For this review, take the finished solid that the model builds, in its own axes (mm). Face numbers are marked on the shaded views. A direction names the side the tool comes from. Give positions to 0.01 mm unless a question says otherwise; leave off trailing zeros. Loops run counter-clockwise (first coordinate to the right, second up) from the corner with the lowest first, then second, coordinate; pieces in that order, holes last. Notation, with made-up numbers: (-21, 22) - (-2, 22) arc R3 ccw to (-2, 26) - close; hole circle Ø7 at (-38, -37.75). An arc over 180 degrees is marked (long way). Answer as CSV lines item,"result".
from build123d import *

# Parameters (mm, degrees)
F0_W      = 50
F0_H      = 30
F1_DEPTH  = 40
F2_W      = 10
F2_H      = 23
F3_DEPTH  = 40.001
F5_DEPTH  = 7.001
F7_DEPTH  = 40.001
F8_DEPTH  = 91
F10_DEPTH = 40.001


# Not quite as in the source:
# - an extrude ends at something that could not be found from the text; its depth is read off the source's solid


with BuildPart() as f1:
    # F0 (on Front) → F1 (new body)
    with BuildSketch(Plane.XZ):
        Rectangle(F0_W, F0_H)
    extrude(amount=F1_DEPTH)

    # F2 (on face) → F3 (cut, through all)
    with BuildSketch(Plane.XZ.offset(40)):
        with Locations((-20, 3.5)):
            Rectangle(F2_W, F2_H)
        with Locations((20, 3.5)):
            Rectangle(F2_W, F2_H)
    extrude(amount=-F3_DEPTH, mode=Mode.SUBTRACT)

    # F4 (on face) → F5 (cut, through all)
    with BuildSketch(Plane.XY.offset(-8)):
        with BuildLine():
            Line((-17.1079541888, -29.1274278762), (-16.9848898668, -10.886759475))
            ThreePointArc((-16.9848898668, -10.886759475), (-20.2301216242, -8.0087862495), (-23, -11.346754618))
            Line((-23, -11.346754618), (-22.9528288916, -29.3672662228))
            ThreePointArc((-22.9528288916, -29.3672662228), (-19.9160668858, -32.0334456443), (-17.1079541888, -29.1274278762))
        make_face()
        with BuildLine():
            ThreePointArc((23, -11.346754618), (20.2301216242, -8.0087862495), (16.9848898668, -10.886759475))
            Line((16.9848898668, -10.886759475), (17.1079541888, -29.1274278762))
            ThreePointArc((17.1079541888, -29.1274278762), (19.9160668858, -32.0334456443), (22.9528288916, -29.3672662228))
            Line((22.9528288916, -29.3672662228), (23, -11.346754618))
        make_face()
    extrude(amount=-F5_DEPTH, mode=Mode.SUBTRACT)

    # F6 (on face) → F7 (cut, through all)
    with BuildSketch(Plane.XZ.offset(40)):
        Polygon((15, 15), (10, 15), (15, -8), align=None)
        Polygon((-15, -8), (-10, 15), (-15, 15), align=None)
    extrude(amount=-F7_DEPTH, mode=Mode.SUBTRACT)

    # F6 (on face) → F8 (cut, through all)
    with BuildSketch(Plane.XZ.offset(40)):
        Polygon((-15, -8), (-10, 15), (-15, 15), align=None)
        Polygon((15, 15), (10, 15), (15, -8), align=None)
    extrude(amount=F8_DEPTH, mode=Mode.SUBTRACT)

    # F9 (on face) → F10 (cut, through all)
    with BuildSketch(Plane.XZ.offset(40)):
        Polygon((-5, 15), (-10, 6.486502476), (0, 6.486502476), (10, 6.486502476), (5, 15), align=None)
    extrude(amount=-F10_DEPTH, mode=Mode.SUBTRACT)


solid = f1.part
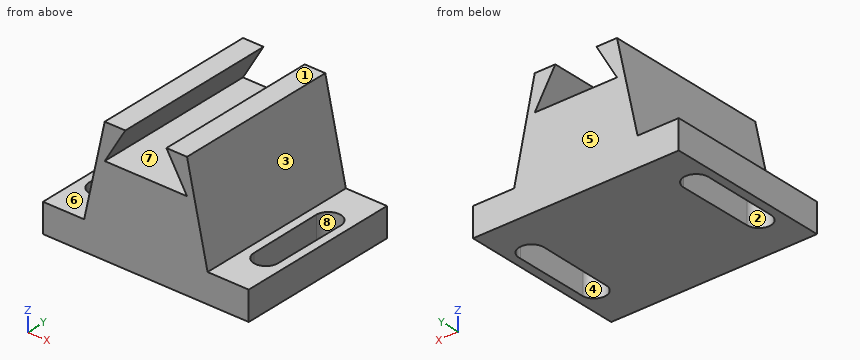
1) Draft analysis for pull direction X (two halves, no side actions). For the marked faces 1, 2, 3 and 4, state which applies: pulls with the +X half, pulls with the -X half, needs draft (parallel to the pull), parting line crosses it, or undercut.
From the geometry:
face 1,"needs draft"
face 2,"undercut"
face 3,"pulls with the +X half"
face 4,"undercut"
2) Consider section D-D on y = -4.5. Write out the cut boundary in (x, z), and give its area (3 significant figures).
From the geometry:
outline,"(-25, -15) - (25, -15) - (25, -8) - (15, -8) - (10, 15) - (5, 15) - (10, 6.49) - (-10, 6.49) - (-5, 15) - (-10, 15) - (-15, -8) - (-25, -8) - close"
area,"797 mm^2"
3) Insertion check: P1, Ø2, axis at y = -22.5, z = 11, coming from the +X side; P2, Ø1.5, axis at x = 17.5, y = -7, coming from the +Z side; P3, Ø4, axis at y = -21, z = -5, coming from the +X side. Each pin has a flat end and moves straight along its axis. Give the tip position at first contact, or say it passes through.
From the geometry:
P1,"stops at x = 11.09"
P2,"stops at z = -8"
P3,"stops at x = 14.78"
4) Consider section B-B on y = -27. Write out the cut boundary in (x, z).
From the geometry:
outline,"(-25, -15) - (-22.96, -15) - (-22.96, -8) - (-25, -8) - close; (-17.09, -15) - (17.09, -15) - (17.09, -8) - (15, -8) - (10, 15) - (5, 15) - (10, 6.49) - (-10, 6.49) - (-5, 15) - (-10, 15) - (-15, -8) - (-17.09, -8) - close; (22.96, -15) - (25, -15) - (25, -8) - (22.96, -8) - close"
5) Consider section C-C on z = 13. Write out the cut boundary in (x, y), and give its area (3 significant figures).
From the geometry:
outline,"(-10.43, -40) - (-6.17, -40) - (-6.17, 0) - (-10.43, 0) - close; (6.17, -40) - (10.43, -40) - (10.43, 0) - (6.17, 0) - close"
area,"341 mm^2"
6) Machinability: for the marked faces 5, 6, 7 and 8, which of the approach directions +Z, -Z, +X, -X, +Y, -Y give a long, thin tool a straight path to every point of the face, cutting with its end or side? Answer none if there is none.
From the geometry:
face 5,"+Z, -Z, +X, -X, +Y"
face 6,"+Z, -X, +Y, -Y"
face 7,"+Y, -Y"
face 8,"+Z, -Z"
7) Wall thickness on line 1 (X direction, y = -31, z = -13); line 2 (Z direction, x = 2, y = -28); line 3 (Z direction, x = -8, y = -15): over which ranges is each line inside the solid? List them lowest first. Write a range as from..to.
From the geometry:
line 1,"x = -25..-22.27, -17.8..17.8, 22.27..25"
line 2,"z = -15..6.49"
line 3,"z = -15..6.49, 9.89..15"
8) Consider section A-A on x = -20. Write out the cut boundary in (y, z), and give its area (3 significant figures).
From the geometry:
outline,"(-40, -15) - (-32.04, -15) - (-32.04, -8) - (-40, -8) - close; (-8, -15) - (0, -15) - (0, -8) - (-8, -8) - close"
area,"112 mm^2"
